from build123d import *

# Parameters (mm, degrees)
SKETCH1_R           = 75
BOSS_EXTRUDE1_DEPTH = 2.5
SKETCH2_R           = 22.5
BOSS_EXTRUDE2_DEPTH = 17.5
SKETCH3_R           = 13
CUT_EXTRUDE1_DEPTH  = 35
CUT_EXTRUDE2_DEPTH  = 35
CUT_EXTRUDE3_DEPTH  = 35
CHAMFER1_SIZE       = 1
FILLET1_R           = 3
CHAMFER2_SIZE       = 1


with BuildPart() as part:
    # Sketch1 → Boss-Extrude1 (new, symmetric)
    with BuildSketch(Plane.XY):
        Circle(SKETCH1_R)
    extrude(amount=BOSS_EXTRUDE1_DEPTH, both=True)

    # Sketch2 → Boss-Extrude2 (add, symmetric)
    with BuildSketch(Plane.XY):
        Circle(SKETCH2_R)
    extrude(amount=BOSS_EXTRUDE2_DEPTH, both=True)

    # Sketch3 → Cut-Extrude1 (cut)
    with BuildSketch(Plane.XY.offset(17.5)):
        Circle(SKETCH3_R)
    extrude(amount=-CUT_EXTRUDE1_DEPTH, mode=Mode.SUBTRACT)

    # Sketch4 → Cut-Extrude2 (cut)
    with BuildSketch(Plane.XY.offset(2.5)):
        with BuildLine():
            ThreePointArc((58.530203334, 46.895791897), (37.5, 64.951905284), (11.347845446, 74.136538925))
            ThreePointArc((11.347845446, 74.136538925), (30, 51.961524227), (58.530203334, 46.895791897))
        make_face()
        with BuildLine():
            ThreePointArc((67.850984929, 31.956906049), (64.951905284, 37.5), (61.600984929, 42.782223596))
            Line((61.600984929, 42.782223596), (31.516016151, 25.412658774))
            ThreePointArc((31.516016151, 25.412658774), (29.228357378, 16.875), (37.766016151, 14.587341226))
            Line((37.766016151, 14.587341226), (67.850984929, 31.956906049))
        make_face()
        with BuildLine():
            ThreePointArc((75, 0), (73.708390494, 13.85904653), (69.87804878, 27.240747028))
            ThreePointArc((69.87804878, 27.240747028), (60, 0), (69.87804878, -27.240747028))
            ThreePointArc((69.87804878, -27.240747028), (73.708390494, -13.85904653), (75, 0))
        make_face()
        with BuildLine():
            ThreePointArc((61.600984929, -42.782223596), (64.951905284, -37.5), (67.850984929, -31.956906049))
            Line((67.850984929, -31.956906049), (37.766016151, -14.587341226))
            ThreePointArc((37.766016151, -14.587341226), (29.228357378, -16.875), (31.516016151, -25.412658774))
            Line((31.516016151, -25.412658774), (61.600984929, -42.782223596))
        make_face()
        with BuildLine():
            ThreePointArc((11.347845446, -74.136538925), (37.5, -64.951905284), (58.530203334, -46.895791897))
            ThreePointArc((58.530203334, -46.895791897), (30, -51.961524227), (11.347845446, -74.136538925))
        make_face()
        with BuildLine():
            Line((-6.25, -40), (-6.25, -74.739129644))
            ThreePointArc((-6.25, -74.739129644), (0, -75), (6.25, -74.739129644))
            Line((6.25, -74.739129644), (6.25, -40))
            ThreePointArc((6.25, -40), (0, -33.75), (-6.25, -40))
        make_face()
        with BuildLine():
            ThreePointArc((-11.347845446, -74.136538925), (-30, -51.961524227), (-58.530203334, -46.895791897))
            ThreePointArc((-58.530203334, -46.895791897), (-37.5, -64.951905284), (-11.347845446, -74.136538925))
        make_face()
        with BuildLine():
            Line((-37.766016151, -14.587341226), (-67.850984929, -31.956906049))
            ThreePointArc((-67.850984929, -31.956906049), (-64.951905284, -37.5), (-61.600984929, -42.782223596))
            Line((-61.600984929, -42.782223596), (-31.516016151, -25.412658774))
            ThreePointArc((-31.516016151, -25.412658774), (-29.228357378, -16.875), (-37.766016151, -14.587341226))
        make_face()
        with BuildLine():
            ThreePointArc((-69.87804878, -27.240747028), (-60, 0), (-69.87804878, 27.240747028))
            ThreePointArc((-69.87804878, 27.240747028), (-75, 0), (-69.87804878, -27.240747028))
        make_face()
        with BuildLine():
            Line((-31.516016151, 25.412658774), (-61.600984929, 42.782223596))
            ThreePointArc((-61.600984929, 42.782223596), (-64.951905284, 37.5), (-67.850984929, 31.956906049))
            Line((-67.850984929, 31.956906049), (-37.766016151, 14.587341226))
            ThreePointArc((-37.766016151, 14.587341226), (-29.228357378, 16.875), (-31.516016151, 25.412658774))
        make_face()
        with BuildLine():
            ThreePointArc((-58.530203334, 46.895791897), (-30, 51.961524227), (-11.347845446, 74.136538925))
            ThreePointArc((-11.347845446, 74.136538925), (-37.5, 64.951905284), (-58.530203334, 46.895791897))
        make_face()
        with BuildLine():
            Line((-6.25, 74.739129644), (-6.25, 40))
            ThreePointArc((-6.25, 40), (0, 33.75), (6.25, 40))
            Line((6.25, 40), (6.25, 74.739129644))
            ThreePointArc((6.25, 74.739129644), (0, 75), (-6.25, 74.739129644))
        make_face()
    extrude(amount=-CUT_EXTRUDE2_DEPTH, mode=Mode.SUBTRACT)

    # Sketch5 → Cut-Extrude3 (cut)
    with BuildSketch(Plane.XY.offset(17.5)):
        with BuildLine():
            Line((-4, 12.369316877), (-4, 15.669316877))
            Line((-4, 15.669316877), (4, 15.669316877))
            Line((4, 15.669316877), (4, 12.369316877))
            ThreePointArc((4, 12.369316877), (0, 13), (-4, 12.369316877))
        make_face()
    extrude(amount=-CUT_EXTRUDE3_DEPTH, mode=Mode.SUBTRACT)

    # Chamfer1
    chamfer1_edges = [part.edges().sort_by_distance(p)[0] for p in [
        (-22.5, 0, 17.5),
    ]]
    chamfer(chamfer1_edges, length=CHAMFER1_SIZE)

    # Fillet1
    fillet1_edges = [part.edges().sort_by_distance(p)[0] for p in [
        (-22.5, 0, -2.5),
        (-22.5, 0, 2.5),
    ]]
    fillet(fillet1_edges, radius=FILLET1_R)

    # Chamfer2
    chamfer2_edges = [part.edges().sort_by_distance(p)[0] for p in [
        (-22.5, 0, -17.5),
    ]]
    chamfer(chamfer2_edges, length=CHAMFER2_SIZE)


solid = part.part
CAD build for the part. Positions are in the model's coordinates, mm. A direction names the side the tool comes from. Round coordinates to 2 decimals unless told otherwise and drop trailing zeros. Loops run counter-clockwise (first coordinate to the right, second up) from the corner with the lowest first, then second, coordinate; pieces in that order, holes last.
(1) Cut at D-D (y = -61.5). Give the cut face in (x, z).
(2) Cut at B-B (x = -47). Give the cut face in (y, z), plus the area to 3 significant figures.
(3) Cut at C-C (z = -8.5). Give the cut face in (x, y).
(4) Cut at A-A (y = 0). Give the cut face in (x, z), plus the area to 3 significant figures.
(5) Wall check: line 1 along Y through (x, z) = (0, 6); line 2 along X through (y, z) = (0, -2); line 3 along Y through (x, z) = (0, -1). Give the ranges that are in metal, low to high.
(6) Two-plate mould, pull along Y, no slides. Class faces 1 (the flat face through (30, 1, 2.5)), 2 (the cylindrical face through (8.768, -74.486, 0.035)), 3 (the flat face through (52.6, 23.15, 0.04)), 4 (the cylindrical face through (-30.36, 51.756, 0.035)): +Y half, -Y half, draft (parallel to the pull), parting line (faces both ways), or undercut.
(7) Drop flat-ended pins along their axis: pin 1 (6 mm diameter, centred on x = 25.5, y = 52.5, fed in from +Z); pin 2 (1 mm diameter, centred on y = -13.5, z = 7, fed in from +X); pin 3 (4 mm diameter, centred on x = 1.5, z = 0, fed in from -Y). Give the stop position or say it passes through.
(8) Which spindle directions (+Z, -Z, +X, -X, +Y, -Y) get a long thin tool onto all of the face, cutting with end or side? Do faces 5 (the flat face through (46.77, 34.22, 0.04)), 6 (the cylindrical face through (8.84, 74.477, 0.035)), 7 (the flat face through (30, 1, -2.5)). Say none if no direction does.
Findings below:
1. outline: (-18.65, -2.5) - (-6.25, -2.5) - (-6.25, 2.5) - (-18.65, 2.5) - close; (6.25, -2.5) - (18.65, -2.5) - (18.65, 2.5) - (6.25, 2.5) - close
2. outline: (-46.48, -2.5) - (-34.35, -2.5) - (-34.35, 2.5) - (-46.48, 2.5) - close; (-19.92, -2.5) - (19.92, -2.5) - (19.92, 2.5) - (-19.92, 2.5) - close; (34.35, -2.5) - (46.48, -2.5) - (46.48, 2.5) - (34.35, 2.5) - close
2. area: 320 mm2
3. outline: circle Ø45 at (0, 0); hole (-4, 12.37) arc R13 ccw (long way) to (4, 12.37) - (4, 15.67) - (-4, 15.67) - close
4. outline: (-60, -2.5) - (-25.5, -2.5) arc R3 cw to (-22.5, -5.5) - (-22.5, -16.5) - (-21.5, -17.5) - (-13, -17.5) - (-13, 17.5) - (-21.5, 17.5) - (-22.5, 16.5) - (-22.5, 5.5) arc R3 cw to (-25.5, 2.5) - (-60, 2.5) - close; (13, -17.5) - (21.5, -17.5) - (22.5, -16.5) - (22.5, -5.5) arc R3 cw to (25.5, -2.5) - (60, -2.5) - (60, 2.5) - (25.5, 2.5) arc R3 cw to (22.5, 5.5) - (22.5, 16.5) - (21.5, 17.5) - (13, 17.5) - close
4. area: 1,050 mm2
5. line 1: y = -22.5 to -13, 15.67 to 22.5
5. line 2: x = -60 to -13, 13 to 60
5. line 3: y = -33.75 to -13, 15.67 to 33.75
6. face 1: draft
6. face 2: -Y half
6. face 3: undercut
6. face 4: +Y half
7. pin 1: stops at z = 2.5
7. pin 2: stops at x = 18.36
7. pin 3: stops at y = -34.82
8. face 5: +Z, -Z
8. face 6: +Z, -Z, +X, +Y
8. face 7: -Z
